from build123d import *

# Parameters (mm, degrees)
CROQUIS1_R              = 9.208992718
SALIENTE_EXTRUIR1_DEPTH = 10
CROQUIS2_R              = 30.329695967
CROQUIS2_R_2            = 12.316965918
CORTAR_EXTRUIR1_DEPTH   = 10
CORTAR_EXTRUIR1_TAPER   = 59
CROQUIS3_R              = 29.014091156
CROQUIS3_R_2            = 12.401894161
CORTAR_EXTRUIR2_DEPTH   = 10
CORTAR_EXTRUIR2_DRAFT   = -59


with BuildPart() as part:
    # Croquis1 → Saliente-Extruir1 (new body)
    with BuildSketch(Plane.XY):
        Polygon((-13.322559753, 8.093787843), (-13.670705761, -7.490781268), (-0.348146008, -15.58456911), (13.322559753, -8.093787843), (13.670705761, 7.490781268), (0.348146008, 15.58456911), align=None)
        Circle(CROQUIS1_R, mode=Mode.SUBTRACT)
    extrude(amount=SALIENTE_EXTRUIR1_DEPTH)

    # Croquis2 → Cortar-Extruir1 (cut)
    with BuildSketch(Plane.XY.offset(10)):
        Circle(CROQUIS2_R)
        Circle(CROQUIS2_R_2, mode=Mode.SUBTRACT)
    extrude(amount=-CORTAR_EXTRUIR1_DEPTH, taper=CORTAR_EXTRUIR1_TAPER, mode=Mode.SUBTRACT)


with BuildPart() as cortar_extruir2_tool:
    # Croquis3 → Cortar-Extruir2 (with draft: the straight prism first)
    with BuildSketch(Plane(origin=(0, 0, 0), x_dir=(-1, 0, 0), z_dir=(0, 0, -1))):
        Circle(CROQUIS3_R)
        Circle(CROQUIS3_R_2, mode=Mode.SUBTRACT)
    extrude(amount=-CORTAR_EXTRUIR2_DEPTH)
    # Cortar-Extruir2: the draft: its side faces are tilted about the plane it starts from
    cortar_extruir2_sides = [cortar_extruir2_tool.faces().sort_by_distance(p)[0] for p in [
        (29.014091156, 0, 5),
        (12.401894161, 0, 5),
    ]]
    draft(cortar_extruir2_sides, Plane(origin=(0, 0, 0), x_dir=(-1, 0, 0), z_dir=(0, 0, -1)), CORTAR_EXTRUIR2_DRAFT)


with BuildPart() as part_1:
    add(part.part)

    # Cortar-Extruir2: cut by cortar_extruir2_tool
    add(cortar_extruir2_tool.part, mode=Mode.SUBTRACT)


solid = part_1.part
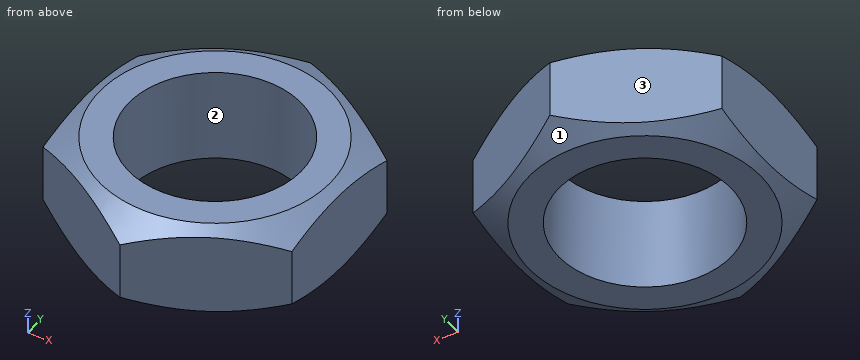
Design review of the part built by this model. Coordinates are the model's own, in mm. Face numbers are marked on the shaded views. Give positions to 0.01 mm unless a question says otherwise; leave off trailing zeros. Write each loop counter-clockwise with the first axis right and the second up, starting at its lowest first coordinate (ties: lowest second). Pieces come first, ordered by that corner, then holes. Notation, with made-up numbers: M 80.5,-17.75 L 127.5,-17.75 A30 ccw 127.5,14.25 Z; hole C 64,79 d1. An arc over 180 degrees is marked long. Return JSON: item names as keys, results as strings. Group by question number.
Item 1: The part is to be moulded in two halves that separate along Y. For the marked faces 1, 2 and 3, say which applies: pulls with the +Y half, pulls with the -Y half, needs draft (parallel to the pull), parting line crosses it, or undercut.
Item 2: Take a section at B-B (x = 0). Give the boundary of the cut face in (y, z).
Item 3: Clearance check with flat-ended pins moving along their axes: pin 1 Ø5 at (y, z) = (-12, 4.5) entering from -X; pin 2 Ø3 at (x, y) = (-6, -1) entering from -Z; pin 3 Ø1.5 at (x, y) = (7.5, 12) entering from -Z. State where each tip first meets the part, or that it passes through.
Item 4: Take a section at A-A (z = 4.5). Give the boundary of the cut face in (x, y), plus the area to 3 significant figures.
Item 5: Wall thickness on line 1 along Y through (x, z) = (6.75, 3.75); line 2 along X through (y, z) = (8.5, 1.25); line 3 along Y through (x, z) = (-2.5, 4.5): over which ranges is each line inside the solid? List them lowest first.
Return value:
{
 "1": {"face 1": "parting line crosses it", "face 2": "undercut", "face 3": "pulls with the +Y half"},
 "2": {"outline": "M -15.39,1.8 L -12.4,0 L -9.21,0 L -9.21,10 L -12.32,10 L -15.39,8.15 Z; M 9.21,0 L 12.4,0 L 15.39,1.8 L 15.39,8.15 L 12.32,10 L 9.21,10 Z"},
 "3": {"pin 1": "stops at x = -10.36", "pin 2": "passes through", "pin 3": "stops at z = 0.6"},
 "4": {"outline": "M -13.67,-7.49 L -0.35,-15.58 L 13.32,-8.09 L 13.67,7.49 L 0.35,15.58 L -13.32,8.09 Z; hole C 0,0 d18.42", "area": "365 mm2"},
 "5": {"line 1": "y = -11.7 to -6.26, 6.26 to 11.7", "line 2": "x = -11.73 to -3.54, 3.54 to 11.73", "line 3": "y = -14.28 to -8.86, 8.86 to 14.02"}
}
